Input: part model. Units: mm. Frame: model coordinates. A direction names the side the tool comes from. Coordinates: 2 decimals unless noted, no trailing zeros. Write each loop counter-clockwise with the first axis right and the second up, starting at its lowest first coordinate (ties: lowest second). Pieces come first, ordered by that corner, then holes. Notation, with made-up numbers: (-18.75, -7.75) - (25.25, -7.75) arc R18 ccw to (25.25, 2.25) - close; hole circle Ø9 at (13, 76.5). An arc over 180 degrees is marked (long way). One line per question, with ' | ' between items. Start each with the question number.
1) Draft query along X for faces 5 (the flat face through (-75, -38.089, 154)), 6 (the cylindrical face through (-126.99, 2.28, 74.58)), 7 (the cylindrical face through (-23.77, 6.76, 94.21)). Return one class per face: released by +X, released by -X, zero draft, split by the parting line, or undercut.
2) First-contact query: P1, Ø6, axis at y = 0, z = 204.48, coming from the +X side; P2, Ø3, axis at y = -24, z = 235.5, coming from the -X side; P3, Ø6, axis at x = -91.5, y = 14, coming from the -Z side. Flat tips, straight axial feed; report the tip coordinate or a pass-through.
3) Section query D-D on x = 0. Return loops of the section in (y, z), and give its area (3 significant figures).
4) Section query A-A on z = 171.5. Return loops of the section in (x, y), and give its area (3 significant figures).
5) Section query B-B on x = -68.5. Return loops of the section in (y, z).
6) Line query: line 1 (Z direction, x = 20.5, y = 2); line 2 (X direction, y = 31, z = 147); line 3 (Z direction, x = -40, y = 20.5). Output: solid intervals per line, ascending.
7) Reachability of faces 1 (the cylindrical face through (-126.99, 2.86, 235.38)), 2 (the cylindrical face through (23.57, -6.08, 94.78)), 3 (the flat face through (-75, 3, 71.733)), 4 (the cylindrical face through (-24.608, -0.22, 81.845)) from +Z, -Z, +X, -X, +Y, -Y: full face, straight path, thin tool, end or side. Return the list, or none.
8) Section query C-C on y = 0. Give the number of separate pieces and of enclosed holes in the cut face, and give its area (3 significant figures).
```python
from build123d import *

# Parameters (mm, degrees)
SZKIC1_R                    = 20
DODANIE_WYCI_GNI_CIE1_DEPTH = 300
SZKIC2_R                    = 10
SZKIC2_R_2                  = 5
DODANIE_WYCI_GNI_CIE2_DEPTH = 30
DODANIE_WYCI_GNI_CIE3_DEPTH = 100
ZAOKR_GLENIE1_R             = 10
ZAOKR_GLENIE2_R             = 2


with BuildPart() as part:
    # Szkic1 → Dodanie-wyciągnięcie1 (new body)
    with BuildSketch(Plane.XY):
        Circle(SZKIC1_R)
    extrude(amount=DODANIE_WYCI_GNI_CIE1_DEPTH)

    # Szkic2 → Dodanie-wyciągnięcie2 (add)
    # profile 1 of 2: a face of its own
    with BuildSketch(Plane(origin=(0, 0, 0), x_dir=(0, 0, -1), z_dir=(1, 0, 0))):
        with Locations((-204.481584116, 0)):
            Circle(SZKIC2_R)
        with Locations(Location((-204.481584116, 0, 0), (0, 0, 180))):
            Circle(SZKIC2_R_2, mode=Mode.SUBTRACT)
    # profile 2 of 2: a face of its own
    with BuildSketch(Plane(origin=(0, 0, 0), x_dir=(0, 0, -1), z_dir=(1, 0, 0))):
        with Locations((-86.839933458, 0)):
            Circle(SZKIC2_R)
        with Locations(Location((-86.839933458, 0, 0), (0, 0, 180))):
            Circle(SZKIC2_R_2, mode=Mode.SUBTRACT)
    dodanie_wyci_gni_cie2 = extrude(amount=DODANIE_WYCI_GNI_CIE2_DEPTH)

    # Lustro1: Dodanie-wyciągnięcie2 across plane
    add(dodanie_wyci_gni_cie2.mirror(Plane(origin=(0, 0, 0), x_dir=(0, 0, 1), z_dir=(1, 0, 0))))

    # Szkic3 → Dodanie-wyciągnięcie3 (add)
    with BuildSketch(Plane.ZY.offset(30)):
        with BuildLine():
            Line((91.732945532, -38.08889509), (218.231237994, -38.08889509))
            ThreePointArc((218.231237994, -38.08889509), (232.373373618, -32.231030714), (238.231237994, -18.08889509))
            Line((238.231237994, -18.08889509), (238.231237994, 23.231699491))
            ThreePointArc((238.231237994, 23.231699491), (232.373373618, 37.373835114), (218.231237994, 43.231699491))
            Line((218.231237994, 43.231699491), (91.732945532, 43.231699491))
            ThreePointArc((91.732945532, 43.231699491), (77.590809908, 37.373835114), (71.732945532, 23.231699491))
            Line((71.732945532, 23.231699491), (71.732945532, -18.08889509))
            ThreePointArc((71.732945532, -18.08889509), (77.590809908, -32.231030714), (91.732945532, -38.08889509))
        make_face()
    extrude(amount=DODANIE_WYCI_GNI_CIE3_DEPTH)

    # Zaokrąglenie1
    zaokr_glenie1_edges = [part.edges().sort_by_distance(p)[0] for p in [
        (-130, -32.231030714, 77.590809908),
        (-130, -38.08889509, 154.982091763),
        (-130, -32.231030714, 232.373373618),
        (-130, 2.5714022, 238.231237994),
        (-130, 37.373835114, 232.373373618),
        (-130, 43.231699491, 154.982091763),
        (-130, 37.373835114, 77.590809908),
        (-130, 2.5714022, 71.732945532),
    ]]
    fillet(zaokr_glenie1_edges, radius=ZAOKR_GLENIE1_R)

    # Zaokrąglenie2
    zaokr_glenie2_edges = [part.edges().sort_by_distance(p)[0] for p in [
        (-30, 0, 214.481584116),
        (-30, 0, 96.839933458),
        (-30, -32.231030714, 77.590809908),
        (-30, -38.08889509, 154.982091763),
        (-30, -32.231030714, 232.373373618),
        (-30, 2.5714022, 238.231237994),
        (-30, 37.373835114, 232.373373618),
        (-30, 43.231699491, 154.982091763),
        (-30, 37.373835114, 77.590809908),
        (-30, 2.5714022, 71.732945532),
    ]]
    fillet(zaokr_glenie2_edges, radius=ZAOKR_GLENIE2_R)


solid = part.part
```
Answer key:
1) face 5: zero draft | face 6: released by -X | face 7: undercut
2) P1: x = 20 | P2: x = -127.38 | P3: z = 71.73
3) outline: (-20, 0) - (20, 0) - (20, 300) - (-20, 300) - close | area: 12,000 mm²
4) outline: (-130, -28.09) arc R10 ccw to (-120, -38.09) - (-32, -38.09) arc R2 ccw to (-30, -36.09) - (-30, 41.23) arc R2 ccw to (-32, 43.23) - (-120, 43.23) arc R10 ccw to (-130, 33.23) - close; circle Ø40 at (0, 0) | area: 9,340 mm²
5) outline: (-38.09, 91.73) arc R20 ccw to (-18.09, 71.73) - (23.23, 71.73) arc R20 ccw to (43.23, 91.73) - (43.23, 218.23) arc R20 ccw to (23.23, 238.23) - (-18.09, 238.23) arc R20 ccw to (-38.09, 218.23) - close
6) line 1: 77.04 to 82.26, 91.42 to 96.64, 194.68 to 199.9, 209.06 to 214.28 | line 2: -130 to -30 | line 3: 71.73 to 238.23
7) face 1: +Z, -X, +Y, -Y | face 2: +X | face 3: -Z, -X, +Y, -Y | face 4: none
8) separate pieces: 1 | enclosed holes: 3 | area: 29,000 mm²
